Geometry check sheet. Reference: the model listing, model coordinates, mm. Face numbers are marked on the shaded views. A direction names the side the tool comes from. Coordinates: 2 decimals unless noted, no trailing zeros. Write each loop counter-clockwise with the first axis right and the second up, starting at its lowest first coordinate (ties: lowest second). Pieces come first, ordered by that corner, then holes. Notation, with made-up numbers: (6, 48.5) -> (39, 48.5) arc R18 cw to (39, 75.5) -> close; hole circle Ø11 at (53.25, 43). An arc over 180 degrees is marked (long way). Answer in a Markdown table with one row per item. Add a question column.
Q1. Section check D-D, the plane x = -8. Record the boundary of the cut face in (y, z).
Q2. Section check C-C, the plane y = 18.25. Record the boundary of the cut face in (x, z) (3 decimals).
Q3. Thickness scan on line 1 (Z direction, x = 7.5, y = 7.75); line 2 (Y direction, x = -6, z = -15); line 3 (X direction, y = 1.75, z = -3). Record the ranges inside material, lowest first.
Q4. Gauge pin test, flat ends, axial feed: P1, Ø12, axis at x = -2, z = -18.5, coming from the +Y side; P2, Ø3, axis at x = -3.5, z = 6, coming from the +Y side. Record the tip position at first contact, or that the pin passes through.
Q5. Section check A-A, the plane x = 10. Record the boundary of the cut face in (y, z) (3 decimals), and give its area (3 significant figures).
Q6. Section check B-B, the plane y = 4.25. Record the boundary of the cut face in (x, z) (3 decimals).
Q7. Tool access check on the marked faces 4 and 5. Record the directions out of +Z, -Z, +X, -X, +Y, -Y that give a thin tool (end or side, any length) a straight path to the whole face; none if there is none.
Q8. Release check for a two-part mould opening along X. For the marked faces 1, 2 and 3 record: pulls with the +X half, pulls with the -X half, needs draft (parallel to the pull), parting line crosses it, or undercut.
```python
from build123d import *

# Parameters (mm, degrees)
SKETCH1_W               = 40
SKETCH1_H               = 48
BOSS_EXTRUDE1_DEPTH     = 9
CUT_EXTRUDE1_DEPTH      = 33.511536414
CUT_EXTRUDE1_DEPTH_BACK = 33.511536414
SKETCH2_R               = 2.625
SKETCH3_R               = 5.75
CUT_EXTRUDE2_DEPTH      = 8
SKETCH5_R               = 3.5
BOSS_EXTRUDE2_DEPTH     = 10
SKETCH6_W               = 40
SKETCH6_H               = 9
BOSS_EXTRUDE3_DEPTH     = 5
CHAMFER1_SIZE           = 10
CUT_EXTRUDE3_DEPTH      = 41.024992192
CUT_EXTRUDE3_DEPTH_BACK = 41.024992192
SKETCH7_R               = 2.125
CUT_EXTRUDE4_START      = -11
SKETCH8_W               = 4.75
SKETCH8_H               = 7.25
SKETCH8_R               = 2.125
CUT_EXTRUDE4_DEPTH      = 11


with BuildPart() as part:
    # Sketch1 → Boss-Extrude1 (new body)
    with BuildSketch(Plane(origin=(0, 0, 0), x_dir=(1, 0, 0), z_dir=(0, 1, 0))):
        Rectangle(SKETCH1_W, SKETCH1_H)
    extrude(amount=BOSS_EXTRUDE1_DEPTH)

    # Sketch2 → Cut-Extrude1 (cut, two sides: drawn at the far end of the back side and taken through both)
    with BuildSketch(Plane.XZ.offset(-CUT_EXTRUDE1_DEPTH_BACK)):
        with Locations(Location((2.5, 0.875, 0), (0, 0, 270))):
            Circle(SKETCH2_R)
    extrude(amount=CUT_EXTRUDE1_DEPTH + CUT_EXTRUDE1_DEPTH_BACK, mode=Mode.SUBTRACT)

    # Sketch3 → Cut-Extrude2 (cut)
    with BuildSketch(Plane(origin=(0, 9, 0), x_dir=(1, 0, 0), z_dir=(0, 1, 0))):
        with Locations(Location((2.5, -0.875, 0), (0, 0, 270))):
            Circle(SKETCH3_R)
    extrude(amount=-CUT_EXTRUDE2_DEPTH, mode=Mode.SUBTRACT)

    # Sketch5 → Boss-Extrude2 (add)
    with BuildSketch(Plane(origin=(0, 9, 0), x_dir=(1, 0, 0), z_dir=(0, 1, 0))):
        with Locations(Location((10, 19, 0), (0, 0, 90))):
            Circle(SKETCH5_R)
    extrude(amount=BOSS_EXTRUDE2_DEPTH)

    # Sketch6 → Boss-Extrude3 (add)
    with BuildSketch(Plane(origin=(0, 0, -24), x_dir=(-1, 0, 0), z_dir=(0, 0, -1))):
        with Locations((0, 4.5)):
            Rectangle(SKETCH6_W, SKETCH6_H)
    extrude(amount=BOSS_EXTRUDE3_DEPTH)

    # Chamfer1
    # the kernel refuses this chamfer: 10 mm, written as the material it adds along each edge
    with BuildSketch(Plane(origin=(10, 9, -19), x_dir=(0, 0, -1), z_dir=(1, 0, 0))) as chamfer1_piece_1_section:
        Polygon((3.5 + CHAMFER1_SIZE, 0), (3.5, CHAMFER1_SIZE), (3.5, 0), align=None)
    chamfer1_piece_1 = revolve(axis=Axis((10, 9, -19), (0, 1, 0)), mode=Mode.PRIVATE)
    chamfer1_piece_1 = split(chamfer1_piece_1, bisect_by=Plane(origin=(20, 13.766694853, -10.450462434), z_dir=(-1, 0, 0)), keep=Keep.TOP, mode=Mode.PRIVATE)
    chamfer1_piece_1 = split(chamfer1_piece_1, bisect_by=Plane(origin=(10, 13.766694853, -29), z_dir=(0, 0, 1)), keep=Keep.TOP, mode=Mode.PRIVATE)
    chamfer1_piece_1 = split(chamfer1_piece_1, bisect_by=Plane(origin=(10, 19, -10.450462434), z_dir=(0, -1, 0)), keep=Keep.TOP, mode=Mode.PRIVATE)
    add(chamfer1_piece_1)

    # Sketch7 → Cut-Extrude3 (cut, two sides: drawn at the far end of the back side and taken through both)
    with BuildSketch(Plane(origin=(0, 19, 0), x_dir=(1, 0, 0), z_dir=(0, 1, 0)).offset(-CUT_EXTRUDE3_DEPTH_BACK)):
        with Locations(Location((10, 19, 0), (0, 0, 270))):
            Circle(SKETCH7_R)
    extrude(amount=CUT_EXTRUDE3_DEPTH + CUT_EXTRUDE3_DEPTH_BACK, mode=Mode.SUBTRACT)

    # Sketch8 → Cut-Extrude4 (cut)
    # profile 1 of 3: a face of its own
    with BuildSketch(Plane.XZ.offset(CUT_EXTRUDE4_START)):
        with Locations((10, -19)):
            Rectangle(SKETCH8_W, SKETCH8_H)
        with Locations(Location((10, -19, 0), (0, 0, 90))):
            Circle(SKETCH8_R, mode=Mode.SUBTRACT)
    # profile 2 of 3: a face of its own
    with BuildSketch(Plane.XZ.offset(CUT_EXTRUDE4_START)):
        Polygon((7.625, -22.625), (7.625, -15.375), (5.532105274, -19), align=None)
    # profile 3 of 3: a face of its own
    with BuildSketch(Plane.XZ.offset(CUT_EXTRUDE4_START)):
        Polygon((14.467894726, -19), (12.375, -22.625), (12.375, -15.375), align=None)
    extrude(amount=CUT_EXTRUDE4_DEPTH, mode=Mode.SUBTRACT)


solid = part.part
```
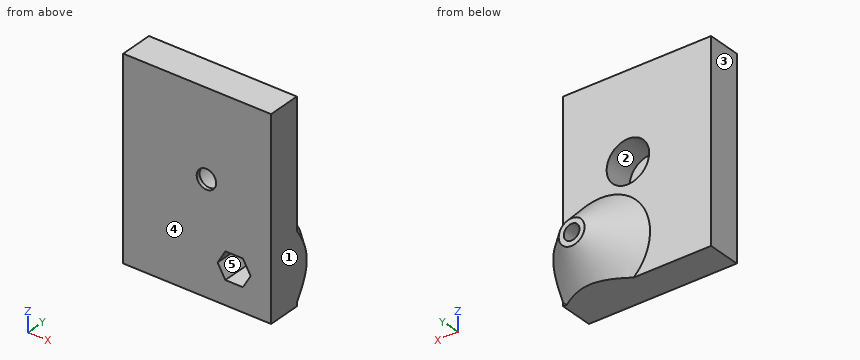
Calculated:
| question | item | result |
|---|---|---|
| 1 | outline | (0, -29) -> (9, -29) -> (9, 24) -> (0, 24) -> close |
| 2 | outline | circle Ø8.5 at (10, -19); hole circle Ø4.25 at (10, -19) |
| 3 | line 1 | z = -29 to -22.41, -15.59 to -1.96, 3.71 to 24 |
| 3 | line 2 | y = 0 to 9 |
| 3 | line 3 | x = -20 to -1.75, 6.75 to 20 |
| 4 | P1 | stops at y = 16.49 |
| 4 | P2 | stops at y = 9 |
| 5 | outline | (0, -29) -> (12.5, -29) -> (19, -22.5) -> (19, -21.125) -> (11, -21.125) -> (11, -22.625) -> (0, -22.625) -> close; (0, -15.375) -> (11, -15.375) -> (11, -16.875) -> (19, -16.875) -> (19, -15.5) -> (9, -5.5) -> (9, 24) -> (0, 24) -> close |
| 5 | area | 527 mm² |
| 6 | outline | (-20, -29) -> (20, -29) -> (20, 24) -> (-20, 24) -> close; hole circle Ø11.5 at (2.5, 0.875); hole (5.532, -19) -> (7.625, -22.625) -> (12.375, -22.625) -> (14.468, -19) -> (12.375, -15.375) -> (7.625, -15.375) -> close |
| 7 | face 4 | +Z, -Z, +X, -X, -Y |
| 7 | face 5 | -Y |
| 8 | face 1 | pulls with the +X half |
| 8 | face 2 | undercut |
| 8 | face 3 | pulls with the -X half |
